Could you check a few things on this model? Use its own coordinates, in mm. A direction names the side the tool comes from. Round coordinates to 2 decimals unless told otherwise and drop trailing zeros. Order: outer loops, then holes, each group sorted by start corner. A loop starts at its lowest first (then second) coordinate and runs counter-clockwise, first axis right, second up. Notation, with made-up numbers: (-31.75, 51.25) - (-3.75, 51.25) arc R28 ccw to (-3.75, 71.25) - close; hole circle Ø10 at (-10, 63.5). An arc over 180 degrees is marked (long way). Use one line per item in the form item = value.
from build123d import *

# Parameters (mm, degrees)
SKETCH_1_W          = 156
SKETCH_1_H          = 40
EXTRUDE_1_DEPTH     = 20
SKETCH_2_W          = 40
SKETCH_2_H          = 20
EXTRUDE_2_DEPTH     = 10
SKETCH_3_W          = 40
SKETCH_3_H          = 20
EXTRUDE_3_DEPTH     = 10
SKETCH_4_W          = 10
SKETCH_4_H          = 40
EXTRUDE_4_DEPTH     = 80
SKETCH_5_W          = 10
SKETCH_5_H          = 40
EXTRUDE_5_DEPTH     = 80
SKETCH_6_R          = 5.75
CUT_EXTRUDE_1_DEPTH = 194
SKETCH_7_W          = 40
SKETCH_7_H          = 40
EXTRUDE_6_DEPTH     = 15
SKETCH_8_W          = 40
SKETCH_8_H          = 25
EXTRUDE_7_DEPTH     = 85
SKETCH_9_W          = 23
SKETCH_9_H          = 12.5
CUT_EXTRUDE_2_DEPTH = 43
SKETCH_10_R         = 2.1
CUT_EXTRUDE_3_DEPTH = 43
SKETCH_11_W         = 68
SKETCH_11_H         = 40
EXTRUDE_8_DEPTH     = 15
SKETCH_12_W         = 68
SKETCH_12_H         = 40
EXTRUDE_9_DEPTH     = 15
SKETCH_13_W         = 156
SKETCH_13_H         = 40
CUT_EXTRUDE_4_DEPTH = 10


with BuildPart() as part:
    # Sketch 1 → Extrude 1 (new body)
    with BuildSketch(Plane(origin=(0, 0, 0), x_dir=(1, 0, 0), z_dir=(0, 1, 0))):
        Rectangle(SKETCH_1_W, SKETCH_1_H)
    extrude(amount=EXTRUDE_1_DEPTH)



with BuildPart() as body_2:
    # Sketch 2 → Extrude 2 (new body)
    with BuildSketch(Plane.ZY.offset(78)):
        with Locations((0, 10)):
            Rectangle(SKETCH_2_W, SKETCH_2_H)
    extrude(amount=EXTRUDE_2_DEPTH)


with BuildPart() as body_3:
    # Sketch 3 → Extrude 3 (new body)
    with BuildSketch(Plane(origin=(78, 0, 0), x_dir=(0, 0, -1), z_dir=(1, 0, 0))):
        with Locations((0, 10)):
            Rectangle(SKETCH_3_W, SKETCH_3_H)
    extrude(amount=EXTRUDE_3_DEPTH)


with BuildPart() as part_1:
    add(part.part)

    add(body_2.part)  # Extrude 4 merges body 2
    # Sketch 4 → Extrude 4 (add)
    with BuildSketch(Plane(origin=(0, 20, 0), x_dir=(1, 0, 0), z_dir=(0, 1, 0))):
        with Locations((-83, 0)):
            Rectangle(SKETCH_4_W, SKETCH_4_H)
    extrude(amount=EXTRUDE_4_DEPTH)


    add(body_3.part)  # Extrude 5 merges body 3
    # Sketch 5 → Extrude 5 (add)
    with BuildSketch(Plane(origin=(0, 20, 0), x_dir=(1, 0, 0), z_dir=(0, 1, 0))):
        with Locations((83, 0)):
            Rectangle(SKETCH_5_W, SKETCH_5_H)
    extrude(amount=EXTRUDE_5_DEPTH)

    # Sketch 6 → Cut-Extrude 1 (cut)
    with BuildSketch(Plane.ZY.offset(88)):
        with Locations((0, 84)):
            Circle(SKETCH_6_R)
    extrude(amount=-CUT_EXTRUDE_1_DEPTH, mode=Mode.SUBTRACT)

    # Sketch 7 → Extrude 6 (add)
    with BuildSketch(Plane.XZ):
        Rectangle(SKETCH_7_W, SKETCH_7_H)
    extrude(amount=EXTRUDE_6_DEPTH)

    # Sketch 8 → Extrude 7 (add)
    with BuildSketch(Plane(origin=(0, 0, -20), x_dir=(-1, 0, 0), z_dir=(0, 0, -1))):
        with Locations((0, -2.5)):
            Rectangle(SKETCH_8_W, SKETCH_8_H)
    extrude(amount=EXTRUDE_7_DEPTH)

    # Sketch 9 → Cut-Extrude 2 (cut)
    with BuildSketch(Plane.ZY.offset(20)):
        with Locations((-93.5, 3.75)):
            Rectangle(SKETCH_9_W, SKETCH_9_H)
    extrude(amount=-CUT_EXTRUDE_2_DEPTH, mode=Mode.SUBTRACT)

    # Sketch 10 → Cut-Extrude 3 (cut)
    with BuildSketch(Plane(origin=(0, -2.5, 0), x_dir=(1, 0, 0), z_dir=(0, 1, 0))):
        with Locations(Location((0, 93.5, 0), (0, 0, 270))):
            Circle(SKETCH_10_R)
    extrude(amount=-CUT_EXTRUDE_3_DEPTH, mode=Mode.SUBTRACT)

    # Sketch 11 → Extrude 8 (add)
    with BuildSketch(Plane.XZ):
        with Locations((54, 0)):
            Rectangle(SKETCH_11_W, SKETCH_11_H)
    extrude(amount=EXTRUDE_8_DEPTH)

    # Sketch 12 → Extrude 9 (add)
    with BuildSketch(Plane.XZ):
        with Locations((-54, 0)):
            Rectangle(SKETCH_12_W, SKETCH_12_H)
    extrude(amount=EXTRUDE_9_DEPTH)

    # Sketch 13 → Cut-Extrude 4 (cut)
    with BuildSketch(Plane(origin=(0, 20, 0), x_dir=(1, 0, 0), z_dir=(0, 1, 0))):
        Rectangle(SKETCH_13_W, SKETCH_13_H)
    extrude(amount=-CUT_EXTRUDE_4_DEPTH, mode=Mode.SUBTRACT)


solid = part_1.part
Item 1: I need wall thicknesses on L1, parallel to Y at x = -82, z = 0; L2, parallel to X at y = 21, z = -8.5; L3, parallel to X at y = -11.75, z = -93.5. Which ranges of each line are inside material? Lowest first, please.
Found:
L1 = -15 to 78.25, 89.75 to 100
L2 = -88 to -78, 78 to 88
L3 = -20 to -2.1, 2.1 to 20
Item 2: Imagine slicing it at B-B on y = 84. Please give me the cut outline in (x, z), plus the area to 3 significant figures.
Found:
outline = (-88, -20) - (-78, -20) - (-78, -5.75) - (-88, -5.75) - close; (-88, 5.75) - (-78, 5.75) - (-78, 20) - (-88, 20) - close; (78, -20) - (88, -20) - (88, -5.75) - (78, -5.75) - close; (78, 5.75) - (88, 5.75) - (88, 20) - (78, 20) - close
area = 570 mm2
Item 3: Imagine slicing it at A-A on x = 0. Please give me the cut outline in (y, z).
Found:
outline = (-15, -105) - (-2.5, -105) - (-2.5, -95.6) - (-15, -95.6) - close; (-15, -91.4) - (-2.5, -91.4) - (-2.5, -82) - (10, -82) - (10, 20) - (-15, 20) - close
Item 4: If we mould it in two halves opening along Y, with no side actions, what happens to faces 1 (the face through (83, 100, 0)), 2 (the face through (-13, 9, 20)), 3 (the face through (82.93, 88.85, 3.09))? For each: released by +Y, released by -Y, zero draft, split by the parting line, or undercut.
Found:
face_1 = released by +Y
face_2 = zero draft
face_3 = undercut
Item 5: For faces 4 (the face through (-1, 10, -20)), 5 (the face through (20, -3, -62)), 6 (the face through (0, -2.5, -91)), which set-ups out of +Z, -Z, +X, -X, +Y, -Y let a thin tool reach every point of the face, with its end or its side?
Found:
face_4 = +Z, -Z, +Y
face_5 = -Z, +X, +Y, -Y
face_6 = -Z, +X, -X, +Y
Item 6: Imagine slicing it at C-C on z = 0. Please give me the cut outline in (x, y), plus the area to 3 significant figures.
Found:
outline = (-88, -15) - (88, -15) - (88, 78.25) - (78, 78.25) - (78, 10) - (-78, 10) - (-78, 78.25) - (-88, 78.25) - close; (-88, 89.75) - (-78, 89.75) - (-78, 100) - (-88, 100) - close; (78, 89.75) - (88, 89.75) - (88, 100) - (78, 100) - close
area = 5,970 mm2
Item 7: Will these pins go through, and if not, where does the flat tip stop? P1, Ø7.5, axis at y = -3, z = -53.5, coming from the -X side; P2, Ø11.5, axis at x = -1, z = -90.5, coming from the +Y side; P3, Ø6, axis at x = -2, y = 6.5, coming from the -Z side.
Found:
P1 = -20
P2 = -2.5
P3 = -82
Item 8: Imagine slicing it at D-D on y = 29. Please give me the cut outline in (x, z), plus the area to 3 significant figures.
Found:
outline = (-88, -20) - (-78, -20) - (-78, 20) - (-88, 20) - close; (78, -20) - (88, -20) - (88, 20) - (78, 20) - close
area = 800 mm2
